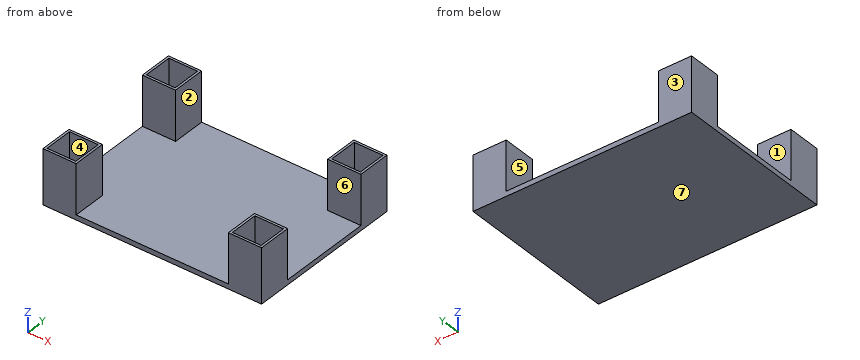
```python
from build123d import *

# Parameters (mm, degrees)
F0_W     = 196.342
F0_H     = 143.764
F1_DEPTH = 4.445
F2_W     = 29.845
F2_H     = 29.845
F2_W_2   = 25.781
F2_H_2   = 25.781
F3_DEPTH = 44.45


with BuildPart() as f1:
    # F0 (on Top) → F1 (new body)
    with BuildSketch(Plane.XY):
        with Locations((9.649968, -21.351978)):
            Rectangle(F0_W, F0_H)
    extrude(amount=F1_DEPTH)

    # F2 (on face) → F3 (join)
    with BuildSketch(Plane.XY.offset(4.445)):
        with Locations((-73.598532, 35.607522)):
            Rectangle(F2_W, F2_H)
        with Locations((-73.598532, 35.607522)):
            Rectangle(F2_W_2, F2_H_2, mode=Mode.SUBTRACT)
        with Locations((92.898468, 35.607522)):
            Rectangle(F2_W, F2_H)
        with Locations((92.898468, 35.607522)):
            Rectangle(F2_W_2, F2_H_2, mode=Mode.SUBTRACT)
        with Locations((92.898468, -78.311478)):
            Rectangle(F2_W, F2_H)
        with Locations((92.898468, -78.311478)):
            Rectangle(F2_W_2, F2_H_2, mode=Mode.SUBTRACT)
        with Locations((-73.598532, -78.311478)):
            Rectangle(F2_W, F2_H)
        with Locations((-73.598532, -78.311478)):
            Rectangle(F2_W_2, F2_H_2, mode=Mode.SUBTRACT)
    extrude(amount=F3_DEPTH)


solid = f1.part
```
Geometry: final body of the model. Coordinates: model frame, mm. Face numbers are marked on the shaded views. A direction names the side the tool comes from. Round coordinates to 2 decimals unless told otherwise and drop trailing zeros. Order: outer loops, then holes, each group sorted by start corner. A loop starts at its lowest first (then second) coordinate and runs counter-clockwise, first axis right, second up. Notation, with made-up numbers: (16, 36) -> (23, 36) arc R14 cw to (23, 63) -> close; hole circle Ø2 at (65, 51.25). An arc over 180 degrees is marked (long way). Write each question's results on one line, items separated by ' | '.
Q1. Pin query (flat end, axial travel): pin 1 Ø2 at (x, y) = (34.5, 35) entering from -Z; pin 2 Ø2 at (x, y) = (10, -42) entering from +Z (3 decimals). Return the tip coordinate at first contact, or that it passes through.
Response values:
pin 1: z = 0 | pin 2: z = 4.445
Q2. Section query B-B (x = 92.5). Output: boundary loops of the cut face in (y, z) (3 decimals), and give its area (3 significant figures).
Response values:
outline: (-93.234, 0) -> (50.53, 0) -> (50.53, 48.895) -> (48.498, 48.895) -> (48.498, 4.445) -> (22.717, 4.445) -> (22.717, 48.895) -> (20.685, 48.895) -> (20.685, 4.445) -> (-63.389, 4.445) -> (-63.389, 48.895) -> (-65.421, 48.895) -> (-65.421, 4.445) -> (-91.202, 4.445) -> (-91.202, 48.895) -> (-93.234, 48.895) -> close | area: 1,000 mm²
Q3. Section query C-C (y = 3). Output: boundary loops of the cut face in (x, z) (3 decimals).
Response values:
outline: (-88.521, 0) -> (107.821, 0) -> (107.821, 4.445) -> (-88.521, 4.445) -> close
Q4. Section query A-A (z = 35). Count the separate pieces of the cut face and the enclosed holes in it, and give its area (3 significant figures).
Response values:
separate pieces: 4 | enclosed holes: 4 | area: 904 mm²
Q5. Access query for the marked faces 4, 5, 6 and 7. Directions: +Z, -Z, +X, -X, +Y, -Y. A direction counts if a zero-diameter tool reaches every point of the face in a straight line with its end or side. Return the directions, or none.
Response values:
face 4: +Z | face 5: +Z, +Y, -Y | face 6: +Z, +X, -X | face 7: -Z, +X, -X, +Y, -Y
Q6. Section query D-D (x = 1.5). Output: boundary loops of the cut face in (y, z) (3 decimals), and give its area (3 significant figures).
Response values:
outline: (-93.234, 0) -> (50.53, 0) -> (50.53, 4.445) -> (-93.234, 4.445) -> close | area: 639 mm²
Q7. Pull-direction query (Y, two-part tool) for the marked faces 1, 2 and 3; classes: released by +Y, released by -Y, zero draft, split by the parting line, or undercut.
Response values:
face 1: undercut | face 2: zero draft | face 3: released by +Y
Q8. Ray query, line 1 along X through (y, z) = (36, 15.5); line 2 along Y through (x, z) = (81, 15); line 3 along X through (y, z) = (22.5, 45.5). Return the intervals inside material, ascending.
Response values:
line 1: -88.52 to -86.49, -60.71 to -58.68, 77.98 to 80.01, 105.79 to 107.82 | line 2: -93.23 to -91.2, -65.42 to -63.39, 20.69 to 22.72, 48.5 to 50.53 | line 3: -88.52 to -58.68, 77.98 to 107.82
